```python
from build123d import *

# Parameters (mm, degrees)
BOSS_EXTRUDE1_DEPTH = 95.25
SKETCH2_R           = 6.858
CUT_EXTRUDE1_DEPTH  = 17.145
SKETCH3_R           = 6.858
CUT_EXTRUDE2_DEPTH  = 17.145
CUT_EXTRUDE3_DEPTH  = 0.254


with BuildPart() as part:
    # Sketch1 → Boss-Extrude1 (new body)
    with BuildSketch(Plane.XY):
        Polygon((14.664696837, 0), (7.332348419, 12.7), (-7.332348419, 12.7), (-14.664696837, 0), (-7.332348419, -12.7), (7.332348419, -12.7), align=None)
    extrude(amount=BOSS_EXTRUDE1_DEPTH)

    # Sketch2 → Cut-Extrude1 (cut)
    with BuildSketch(Plane.XY.offset(95.25)):
        Circle(SKETCH2_R)
    extrude(amount=-CUT_EXTRUDE1_DEPTH, mode=Mode.SUBTRACT)

    # Sketch3 → Cut-Extrude2 (cut)
    with BuildSketch(Plane(origin=(0, 0, 0), x_dir=(-1, 0, 0), z_dir=(0, 0, -1))):
        Circle(SKETCH3_R)
    extrude(amount=-CUT_EXTRUDE2_DEPTH, mode=Mode.SUBTRACT)

    # Sketch5 → Cut-Extrude3 (cut)
    with BuildSketch(Plane(origin=(0, 12.7, 0), x_dir=(1, 0, 0), z_dir=(0, 1, 0))):
        Polygon((-1.600451542, -71.949067171), (1.600451542, -71.949067171), (1.600451542, -36.866567036), (3.153270171, -36.866567036), (0, -31.40494289), (-3.153270171, -36.866567036), (-1.600451542, -36.866567036), (-1.600451542, -42.196329226), align=None)
    extrude(amount=-CUT_EXTRUDE3_DEPTH, mode=Mode.SUBTRACT)


solid = part.part
```
Geometry: final body of the model. Coordinates: model frame, mm. A direction names the side the tool comes from. Coordinates: 2 decimals unless noted, no trailing zeros. Order: outer loops, then holes, each group sorted by start corner. A loop starts at its lowest first (then second) coordinate and runs counter-clockwise, first axis right, second up. Notation, with made-up numbers: (80.5, 40) - (136.5, 40) arc R18 cw to (136.5, 47) - close; hole circle Ø7 at (-38.5, 29). An arc over 180 degrees is marked (long way). Write each question's results on one line, items separated by ' | '.
(1) Section query C-C, the plane z = 25.5. Return the cut outline in (x, y), plus the area to 3 significant figures.
Values found:
outline: (-14.66, 0) - (-7.33, -12.7) - (7.33, -12.7) - (14.66, 0) - (7.33, 12.7) - (-7.33, 12.7) - close | area: 559 mm²
(2) Section query B-B, the plane y = 3.5. Return the cut outline in (x, z) (3 decimals), plus the area to 3 significant figures.
Values found:
outline: (-12.644, 0) - (-5.898, 0) - (-5.898, 17.145) - (5.898, 17.145) - (5.898, 0) - (12.644, 0) - (12.644, 95.25) - (5.898, 95.25) - (5.898, 78.105) - (-5.898, 78.105) - (-5.898, 95.25) - (-12.644, 95.25) - close | area: 2,000 mm²
(3) Mould query, pull axis Y, two halves, no side actions, for faces 1 (the face through (0, 0, 78.105)), 2 (the face through (6, 6, 95.25)), 3 (the face through (10.947, -6.439, 46.958)). Classes: +Y half, -Y half, draft (parallel to the pull), parting line (faces both ways), or undercut.
Values found:
face 1: undercut | face 2: draft | face 3: -Y half
(4) First-contact query: pin 1 Ø3 at (x, z) = (-11, 69) entering from +Y; pin 2 Ø1.5 at (x, y) = (-1, 5) entering from -Z (3 decimals); pin 3 Ø11 at (x, y) = (0, 0) entering from +Z (3 decimals). Flat tips, straight axial feed; report the tip coordinate or a pass-through.
Values found:
pin 1: stops at y = 8.95 | pin 2: stops at z = 17.145 | pin 3: stops at z = 78.105
(5) Section query D-D, the plane x = -9.25. Return the cut outline in (y, z), plus the area to 3 significant figures.
Values found:
outline: (-9.38, 0) - (9.38, 0) - (9.38, 95.25) - (-9.38, 95.25) - close | area: 1,790 mm²
(6) Section query A-A, the plane z = 43. Return the cut outline in (x, y).
Values found:
outline: (-14.66, 0) - (-7.33, -12.7) - (7.33, -12.7) - (14.66, 0) - (7.33, 12.7) - (1.6, 12.7) - (1.6, 12.45) - (-1.6, 12.45) - (-1.6, 12.7) - (-7.33, 12.7) - close
(7) Line query: line 1 (Y direction, x = 0, z = 83.25); line 2 (Y direction, x = 0.5, z = 32.5); line 3 (X direction, y = 0.75, z = 16). Output: solid intervals per line, ascending. Write a range as [from, to].
Values found:
line 1: y = [-12.7, -6.86], [6.86, 12.7] | line 2: y = [-12.7, 12.45] | line 3: x = [-14.23, -6.82], [6.82, 14.23]
(8) Set-up query: faces 4 (the face through (6, 6, 0)), 5 (the face through (-1.487, -6.695, 86.798)), 6 (the face through (1.487, -6.695, 8.452)). Return all of +Z, -Z, +X, -X, +Y, -Y with unobstructed straight access to the full face (end or side cutting, diameter ignored); none if empty.
Values found:
face 4: -Z, +X, -X, +Y, -Y | face 5: +Z | face 6: -Z
